Part model, mm, in its own coordinate system. Face numbers are marked on the shaded views. A direction names the side the tool comes from. Give positions to 0.01 mm unless a question says otherwise; leave off trailing zeros. Write each loop counter-clockwise with the first axis right and the second up, starting at its lowest first coordinate (ties: lowest second). Pieces come first, ordered by that corner, then holes. Notation, with made-up numbers: M 43.5,-15.75 L 81.5,-15.75 A11 ccw 81.5,-6.75 Z; hole C 84.5,28.25 d9. An arc over 180 degrees is marked long. Write item = value, one per line. Start each with the question number.
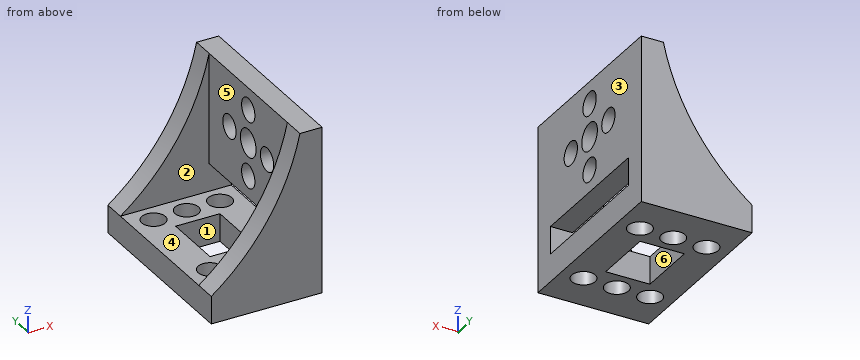
Autodesk Inventor part; units mm, degrees
ref_plane "YZ Plane" through (0, 0, 0) normal (1, 0, 0) x (0, 1, 0)
ref_plane "XZ Plane" through (0, 0, 0) normal (0, 1, 0) x (-1, 0, 0)
ref_plane "XY Plane" through (0, 0, 0) normal (0, 0, 1) x (1, 0, 0)
sketch "Sketch1" plane through (0, 0, 0) normal (0, 1, 0) x (-1, 0, 0)
  circle A0 centre (0, 0) radius 10
  dimension "d0" = 20
extrude "Extrusion1" add sketch "Sketch1" along normal blind 4
sketch "Sketch2" plane through (0, 4, 0) normal (0, 1, 0) x (1, 0, 0)
  line L0 (0, 0) -> (0, 6)
  circle A0 centre (0, 6) radius 2.125
  dimension "d3" = 6
  dimension "d4" = 4.25
extrude "Extrusion2" cut sketch "Sketch2" against normal through all
pattern_circular "Circular Pattern1" count 4 over 360 about axis through (0, 0, 0) along (0, 1, 0) of "Extrusion2"
sketch "Sketch3" plane through (0, 0, 0) normal (0, -1, 0) x (1, 0, 0)
  circle A0 centre (0, 0) radius 10
  arc A1 (-10, 0) -> (10, 0) centre (0, 0) ccw
  line L0 (10, 0) -> (10, -25)
  line L1 (10, -25) -> (-10, -25)
  line L2 (-10, -25) -> (-10, 0)
  dimension "d10" = 25
extrude "Extrusion3" add sketch "Sketch3" against normal blind 4 contours L0 L1 L2 A0
sketch "Sketch4" plane through (0, 4, 0) normal (0, 1, 0) x (1, 0, 0)
  line L0 (-10, 25) -> (-10, 0)
  line L1 (10, 25) -> (-10, 25)
  line L2 (-10, 25) -> (-10, 20)
  line L3 (-10, 20) -> (10, 20)
  line L4 (10, 20) -> (10, 25)
  point P0 (0, 0)
  dimension "d13" = 5
extrude "Extrusion4" add sketch "Sketch4" along normal blind 27
sketch "Sketch5" plane through (10, 0, -25) normal (0, 0, -1) x (-1, 0, 0)
  point P0 (10, 0)
sketch "Sketch6" plane through (10, 0, -25) normal (0, 0, -1) x (-1, 0, 0)
  line L0 (7.875, 4) -> (12.125, 4)
  line L1 (20, 31) -> (0, 31)
  line L2 (10, 17.5) -> (20, 17.5)
  line L3 (10, 17.5) -> (10, 23.5)
  line L4 (10, 23.5) -> (10, 25.5)
  circle A0 centre (10, 25.5) radius 2.125
  point P0 (10, 0)
  dimension "d16" = 6
  dimension "d26" = 2
  dimension "d27" = 4.25
extrude "Extrusion5" cut sketch "Sketch6" against normal through all
pattern_linear "Rectangular Pattern1" count 3 spacing 6 along (-1, 0, 0) count 2 spacing 18 along (0, -1, 0) of "Extrusion5" first direction both ways yes
sketch "Sketch7" plane through (-10, 4, -20) normal (0, 0, 1) x (1, 0, 0)
  circle A0 centre (10, 21.5) radius 2.125
  circle A1 centre (10, 3.5) radius 2.125
  line L0 (10, 21.5) -> (10, 3.5)
  line L1 (6, 7) -> (14, 7)
  line L2 (14, 7) -> (14, 18)
  line L3 (14, 18) -> (6, 18)
  line L4 (6, 18) -> (6, 7)
  line L5 (6, 7) -> (14, 18) construction
  line L6 (14, 7) -> (6, 18) construction
  point P0 (10, -4)
  point P1 (10, 12.5)
  dimension "d29" = 8
  dimension "d30" = 11
extrude "Extrusion6" cut sketch "Sketch7" against normal through all contours L3 L2 L1 L0 | L0 L1 L4 L3
sketch "Sketch8" plane through (-10, 4, -20) normal (0, 0, 1) x (1, 0, 0)
  circle A0 centre (4, 21.5) radius 2.125
  line L0 (4, 21.5) -> (4, 25)
  point P0 (10, -4)
  dimension "d33" = 3.5
sketch "Sketch9" plane through (10, 0, -25) normal (0, 0, -1) x (-1, 0, 0)
  circle A0 centre (16, 25.5) radius 2.125
  line L0 (16, 25.5) -> (16, 29)
  line L1 (20, 4) -> (20, 31)
  line L2 (20, 29) -> (0, 29)
  line L3 (0, 29) -> (0, 33)
  line L4 (0, 33) -> (20, 33)
  line L5 (20, 33) -> (20, 29)
  point P0 (10, 0)
  dimension "d34" = 3.5
  dimension "d35" = 4
extrude "Extrusion7" add sketch "Sketch9" against normal blind 30 contours L2 L3 L4 L5 L1
sketch "Sketch10" plane through (0, 0, 0) normal (0, -1, 0) x (1, 0, 0)
  line L0 (-10, -20) -> (11.4929, -20)
  line L1 (11.4929, -20) -> (11.4929, 11.4929)
  line L2 (11.4929, 11.4929) -> (-10, 11.4929)
  line L3 (-10, 11.4929) -> (-10, -20)
  point P0 (0, 0)
extrude "Extrusion8" cut sketch "Sketch10" against normal blind 4
sketch "Sketch11" plane through (-10, 0, -20) normal (0, 0, 1) x (1, 0, 0)
  line L0 (20, 29) -> (20, 0)
  line L1 (0, 0) -> (20, 0)
  line L2 (20, 0) -> (20, 4)
  line L3 (20, 4) -> (0, 4)
  line L4 (0, 4) -> (0, 0)
  point P0 (10, 0)
  dimension "d40" = 4
extrude "Extrusion9" add sketch "Sketch11" along normal blind 25
sketch "Sketch12" plane through (10, 0, -25) normal (1, 0, 0) x (0, 0, -1)
  line L0 (-5, 29) -> (-30, 29)
  line L1 (-30, 4) -> (-10, 4)
  line L2 (-10, 4) -> (-10, 29)
  line L3 (-10, 29) -> (-30, 29)
  line L4 (-30, 29) -> (-30, 4)
  point P0 (-25, 0)
  dimension "d43" = 20
extrude "Extrusion10" add sketch "Sketch12" against normal blind 4
sketch "Sketch13" plane through (10, 0, 5) normal (1, 0, 0) x (0, 0, -1)
  line L0 (20, 29) -> (20, 4)
  line L1 (20, 16.5) -> (0, 16.5)
  line L2 (0, 0) -> (0, 33)
  line L3 (10, 16.5) -> (4, 16.5)
  circle A0 centre (10, 16.5) radius 2.5
  point P0 (5, 0)
  dimension "d46" = 6
  dimension "d47" = 5
extrude "Extrusion11" cut sketch "Sketch13" against normal through all
sketch "Sketch14" plane through (10, 0, 5) normal (1, 0, 0) x (0, 0, -1)
  circle A0 centre (10, 16.5) radius 2.5
  line L0 (10, 16.5) -> (4, 16.5)
  circle A1 centre (4, 16.5) radius 2.125
  point P0 (5, 0)
  dimension "d50" = 6
  dimension "d51" = 4.25
extrude "Extrusion12" cut sketch "Sketch14" against normal through all contours A1
pattern_circular "Circular Pattern2" count 4 over 360 about axis through (10, 16.5, -5) along (-1, 0, 0) of "Extrusion12"
sketch "Sketch15" plane through (-10, 33, -25) normal (0, 1, 0) x (1, 0, 0)
  line L0 (16, -30) -> (0, -30)
  line L1 (0, -30) -> (16, -30)
  line L2 (0, -30) -> (0, -5)
  line L3 (0, 0) -> (0, -30)
  arc A0 (16, -30) -> (0, -5) centre (-25.4317, -38.8963) ccw
  point P0 (10, -25)
  dimension "d57" = 25
extrude "Extrusion13" cut sketch "Sketch15" against normal through all
properties part number "PickJoint"
Q1. Slice it at B-B (x = 7.25). Give the cut face in (y, z) (3 decimals), and give its area (3 significant figures).
Q2. Probe line 1 along Y through (x, z) = (6, -23.65) (3 decimals); line 2 along X through (y, z) = (7.5, -22) (3 decimals); line 3 along Y through (x, z) = (7.75, -16.5). List the from-to ranges inside material, lowest first.
Q3. Tool access for the marked faces 4, 5 and 6: list every direction of +Z, -Z, +X, -X, +Y, -Y with a clear straight run to the whole face (end or side of a thin tool).
Q4. Slice it at D-D (z = -11). Give the cut face in (x, y) (3 decimals).
Q5. Slice it at A-A (y = 22.5). Give the cut face in (x, z) (3 decimals).
Q6. Drop flat-ended pins along their axis: P1, Ø2.5, axis at x = 0, y = 25.5, coming from the +Z side; P2, Ø5, axis at y = 10.5, z = -5, coming from the -X side. Give the stop position or say it passes through.
Q7. Two-plate mould, pull along X, no slides. Class the marked faces 1, 2 and 3: +X half, -X half, draft (parallel to the pull), parting line (faces both ways), or undercut.
Q8. Slice it at C-C (y = 16.5). Give the cut face in (x, z) (3 decimals).
Working result:
q1.outline = M 0,-25 L 5.782,-25 L 5.782,-20 L 4,-20 L 4,-15 L 29,-15 L 29,-20 L 27.218,-20 L 27.218,-25 L 33,-25 L 33,5 L 0,5 Z; M 9.218,-25 L 23.782,-25 L 23.782,-20 L 9.218,-20 Z; hole C 10.5,-5 d4.25; hole C 16.5,-5 d5; hole C 16.5,-11 d4.25; hole C 16.5,1 d4.25; hole C 22.5,-5 d4.25
q1.area = 754 mm2
q2.line_1 = 0 to 5.375, 9.625 to 23.375, 27.625 to 33
q2.line_2 = -10 to -8.125, -3.875 to -2.125, 2.125 to 3.875, 8.125 to 10
q2.line_3 = 0 to 4, 29 to 33
q3.face_4 = +X, -X
q3.face_5 = +Z, -X
q3.face_6 = +Z, -Z
q4.outline = M -1.14,0 L 10,0 L 10,14.375 L 6,14.375 L 6,4 L -1.14,4 Z; M -1.14,29 L 6,29 L 6,18.625 L 10,18.625 L 10,33 L -1.14,33 Z
q5.outline = M -10,-25 L 10,-25 L 10,-20 L -10,-20 Z; M 6,-15 L 10,-15 L 10,-7.125 L 6,-7.125 Z; M 6,-2.875 L 10,-2.875 L 10,5 L 6,5 Z
q6.P1 = through
q6.P2 = 6
q7.face_1 = undercut
q7.face_2 = draft
q7.face_3 = +X half
q8.outline = M -10,-25 L -4,-25 L -4,-20 L -10,-20 Z; M 4,-25 L 10,-25 L 10,-20 L 4,-20 Z; M 6,-15 L 10,-15 L 10,-13.125 L 6,-13.125 Z; M 6,-8.875 L 10,-8.875 L 10,-7.5 L 6,-7.5 Z; M 6,-2.5 L 10,-2.5 L 10,-1.125 L 6,-1.125 Z; M 6,3.125 L 10,3.125 L 10,5 L 6,5 Z
